from build123d import *

# Parameters (mm, degrees)
SKETCH1_R               = 7.071067812
SKETCH1_R_2             = 3
SKETCH1_W               = 80
SKETCH1_H               = 10
BOSS_EXTRUDE1_DEPTH     = 6
SKETCH2_R               = 3
CUT_EXTRUDE1_DEPTH      = 3
SKETCH3_R               = 2
CUT_EXTRUDE2_DEPTH      = 44.081025369
SKETCH4_R               = 3.5
CUT_EXTRUDE3_DEPTH      = 0.6
CUT_EXTRUDE4_DEPTH      = 24
CUT_EXTRUDE4_DEPTH_BACK = 44.081025369
SKETCH5_R               = 1.5


with BuildPart() as part:
    # Sketch1 → Boss-Extrude1 (new body)
    with BuildSketch(Plane.XY):
        with Locations((-35, 0)):
            Circle(SKETCH1_R)
        with Locations((-35, 0)):
            Circle(SKETCH1_R_2)
        with Locations((35, 0)):
            Circle(SKETCH1_R)
        with Locations((35, 0)):
            Circle(SKETCH1_R_2)
        Rectangle(SKETCH1_W, SKETCH1_H)
    extrude(amount=BOSS_EXTRUDE1_DEPTH)

    # Sketch2 → Cut-Extrude1 (cut)
    with BuildSketch(Plane.XY.offset(6)):
        with Locations((-35, 0)):
            Circle(SKETCH2_R)
        with Locations(Location((35, 0, 0), (0, 0, 180))):
            Circle(SKETCH2_R)
    extrude(amount=-CUT_EXTRUDE1_DEPTH, mode=Mode.SUBTRACT)

    # Sketch3 → Cut-Extrude2 (cut, through all)
    with BuildSketch(Plane.XY.offset(6)):
        with Locations((-35, 0)):
            Circle(SKETCH3_R)
        with Locations(Location((35, 0, 0), (0, 0, 180))):
            Circle(SKETCH3_R)
    extrude(amount=-CUT_EXTRUDE2_DEPTH, mode=Mode.SUBTRACT)

    # Sketch4 → Cut-Extrude3 (cut)
    with BuildSketch(Plane.XY.offset(6)):
        with Locations((-35, 0)):
            Circle(SKETCH4_R)
        with Locations(Location((35, 0, 0), (0, 0, 180))):
            Circle(SKETCH4_R)
    extrude(amount=-CUT_EXTRUDE3_DEPTH, mode=Mode.SUBTRACT)

    # Sketch5 → Cut-Extrude4 (cut, two sides: drawn at the far end of the back side and taken through both)
    with BuildSketch(Plane.XY.offset(6).offset(-CUT_EXTRUDE4_DEPTH_BACK)):
        with Locations(Location((0, 0, 0), (0, 0, 180))):
            Circle(SKETCH5_R)
    extrude(amount=CUT_EXTRUDE4_DEPTH + CUT_EXTRUDE4_DEPTH_BACK, mode=Mode.SUBTRACT)


solid = part.part
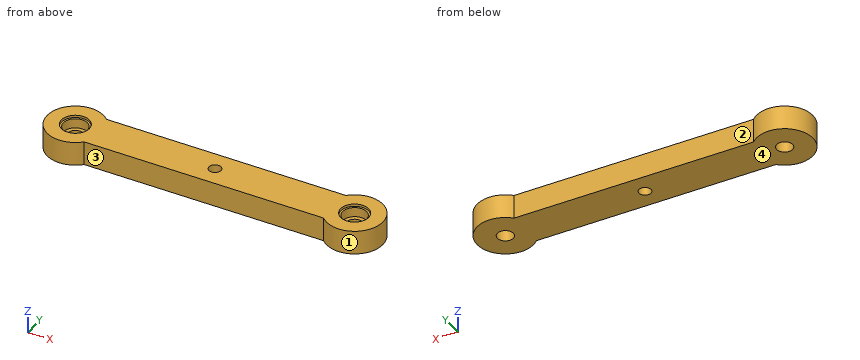
Input: part model. Units: mm. Frame: model coordinates. Face numbers are marked on the shaded views. A direction names the side the tool comes from. Coordinates: 2 decimals unless noted, no trailing zeros. Order: outer loops, then holes, each group sorted by start corner. A loop starts at its lowest first (then second) coordinate and runs counter-clockwise, first axis right, second up.
1. Ray query, line 1 along Y through (x, z) = (0, 4.75); line 2 along Y through (x, z) = (35, 4.2); line 3 along X through (y, z) = (0.25, 3.45). Return the intervals inside material, ascending.
Checked values:
line 1: y = -5 to -1.5, 1.5 to 5
line 2: y = -7.07 to -3, 3 to 7.07
line 3: x = -42.07 to -37.99, -32.01 to -1.48, 1.48 to 32.01, 37.99 to 42.07
2. Cut plane B-B, the plane y = 0. Count the separate pieces of the cut face and the enclosed holes in it, plus the area to 3 significant figures.
Checked values:
separate pieces: 4
enclosed holes: 0
area: 426 mm2
3. Contact query for flat-ended pins moving along their axis: P1, Ø6.5, axis at x = -35, y = 0, coming from the -Z side; P2, Ø1.5, axis at y = -5.5, z = 2, coming from the -X side; P3, Ø1.5, axis at x = -21.5, z = 4.5, coming from the -Y side; P4, Ø6.5, axis at x = -35, y = 0, coming from the +Z side. Output: stop coordinate, or through.
Checked values:
P1: stops at z = 0
P2: stops at x = -40.24
P3: stops at y = -5
P4: stops at z = 5.4
4. Cut plane D-D, the plane y = 6. Return loops of the section in (x, z).
Checked values:
outline: (-38.74, 0) - (-31.26, 0) - (-31.26, 6) - (-38.74, 6) - close; (31.26, 0) - (38.74, 0) - (38.74, 6) - (31.26, 6) - close
5. Access query for the marked faces 1 and 2. Directions: +Z, -Z, +X, -X, +Y, -Y. A direction counts if a zero-diameter tool reaches every point of the face in a straight line with its end or side. Return the directions, or none.
Checked values:
face 1: +Z, -Z
face 2: +Z, -Z, +Y
6. Cut plane C-C, the plane z = 4.55. Return loops of the section in (x, y), plus the area to 3 significant figures.
Checked values:
outline: (-30, -5) - (30, -5) arc R7.07 ccw (long way) to (30, 5) - (-30, 5) arc R7.07 ccw (long way) to start; hole circle Ø6 at (-35, 0); hole circle Ø3 at (0, 0); hole circle Ø6 at (35, 0)
area: 822 mm2
7. Draft query along X for the marked faces 3 and 4. Return one class per face: +X half, -X half, draft (parallel to the pull), parting line (faces both ways), or undercut.
Checked values:
face 3: undercut
face 4: draft
8. Cut plane A-A, the plane x = 0. Return loops of the section in (y, z).
Checked values:
outline: (-5, 0) - (-1.5, 0) - (-1.5, 6) - (-5, 6) - close; (1.5, 0) - (5, 0) - (5, 6) - (1.5, 6) - close
